from build123d import *

# Parameters (mm, degrees)
SKETCH1_W               = 13.75
SKETCH1_H               = 13.75
BASEBOSS_EXTRUDE1_DEPTH = 1
WALLSSKETCH2_W          = 13.75
WALLSSKETCH2_H          = 13.75
WALLSSKETCH2_W_2        = 9.75
WALLSSKETCH2_H_2        = 9.75
BOSS_EXTRUDE2_DEPTH     = 6.5
SKETCH3_W               = 13.75
SKETCH3_H               = 13.75
BOSS_EXTRUDE3_DEPTH     = 2


with BuildPart() as part:
    # Sketch1 → BaseBoss-Extrude1 (new body)
    with BuildSketch(Plane.XY):
        with Locations((6.875, 6.875)):
            Rectangle(SKETCH1_W, SKETCH1_H)
    extrude(amount=BASEBOSS_EXTRUDE1_DEPTH)

    # WallsSketch2 → Boss-Extrude2 (add)
    with BuildSketch(Plane.XY.offset(1)):
        with Locations((6.875, 6.875)):
            Rectangle(WALLSSKETCH2_W, WALLSSKETCH2_H)
        with Locations((6.875, 6.875)):
            Rectangle(WALLSSKETCH2_W_2, WALLSSKETCH2_H_2, mode=Mode.SUBTRACT)
    extrude(amount=BOSS_EXTRUDE2_DEPTH)

    # Sketch3 → Boss-Extrude3 (add)
    with BuildSketch(Plane.XY.offset(7.5)):
        with Locations((6.875, 6.875)):
            Rectangle(SKETCH3_W, SKETCH3_H)
        Polygon((2, 3), (5.623475836, 6.623475836), (4.209262274, 8.037689399), (2, 5.828427125), (2, 11.75), (3, 11.75), (4.767766953, 9.982233047), (6.181980515, 11.396446609), (5.828427125, 11.75), (7.921572875, 11.75), (7.568019485, 11.396446609), (8.982233047, 9.982233047), (10.75, 11.75), (11.75, 11.75), (11.75, 5.828427125), (9.540737726, 8.037689399), (8.126524164, 6.623475836), (11.75, 3), (11.75, 2), (2, 2), align=None, mode=Mode.SUBTRACT)
    extrude(amount=BOSS_EXTRUDE3_DEPTH)


solid = part.part
Input: part model. Units: mm. Frame: model coordinates. A direction names the side the tool comes from. Give positions to 0.01 mm unless a question says otherwise; leave off trailing zeros. Order: outer loops, then holes, each group sorted by start corner. A loop starts at its lowest first (then second) coordinate and runs counter-clockwise, first axis right, second up.
Q1. Section D-D on x = 3.5. Output: boundary loops of the cut face in (y, z), and give its area (3 significant figures).
Checked values:
outline: (0, 0) - (13.75, 0) - (13.75, 9.5) - (11.25, 9.5) - (11.25, 7.5) - (11.75, 7.5) - (11.75, 1) - (2, 1) - (2, 9.5) - (0, 9.5) - close; (4.5, 7.5) - (7.33, 7.5) - (7.33, 9.5) - (4.5, 9.5) - close
area: 54.4 mm2
Q2. Ray query, probe 1 along Y at (x, z) = (11.5, 4.75); probe 2 along Y at (x, z) = (4.5, 8.25). Return the intervals inside material, ascending.
Checked values:
probe 1: y = 0 to 2, 11.75 to 13.75
probe 2: y = 0 to 2, 5.5 to 7.75, 10.25 to 13.75
Q3. Section B-B on x = 7.25. Output: boundary loops of the cut face in (y, z).
Checked values:
outline: (0, 0) - (13.75, 0) - (13.75, 9.5) - (11.75, 9.5) - (11.75, 1) - (2, 1) - (2, 9.5) - (0, 9.5) - close
Q4. Set-up query: faces 1 (the flat face through (10.66, 6.92, 8.49)), 2 (the flat face through (13.75, 7, 5)), 3 (the flat face through (2, 7, 5)). Return all of +Z, -Z, +X, -X, +Y, -Y with unobstructed straight access to the full face (end or side cutting, diameter ignored); none if empty.
Checked values:
face 1: +Z
face 2: +Z, -Z, +X, +Y, -Y
face 3: none
Q5. Draft query along X for faces 4 (the flat face through (5, 7, 9.5)), 5 (the flat face through (0, 7, 5)), 6 (the flat face through (5, 11, 7.5)), 7 (the flat face through (7, 7, 1)). Return one class per face: +X half, -X half, draft (parallel to the pull), parting line (faces both ways), or undercut.
Checked values:
face 4: draft
face 5: -X half
face 6: undercut
face 7: undercut
Q6. Section A-A on z = 3.75. Output: boundary loops of the cut face in (x, y).
Checked values:
outline: (0, 0) - (13.75, 0) - (13.75, 13.75) - (0, 13.75) - close; hole (2, 2) - (11.75, 2) - (11.75, 11.75) - (2, 11.75) - close
Q7. Section C-C on y = 4.5. Output: boundary loops of the cut face in (x, z), and give its area (4 significant figures).
Checked values:
outline: (0, 0) - (13.75, 0) - (13.75, 9.5) - (10.25, 9.5) - (10.25, 7.5) - (11.75, 7.5) - (11.75, 1) - (2, 1) - (2, 7.5) - (3.5, 7.5) - (3.5, 9.5) - (0, 9.5) - close
area: 53.75 mm2
